Can you work these out from the model? Positions are in its coordinate system, mm. A direction names the side the tool comes from. Coordinates: 2 decimals unless noted, no trailing zeros. Write each loop counter-clockwise with the first axis right and the second up, starting at its lowest first coordinate (ties: lowest second). Pieces come first, ordered by that corner, then holes. Notation, with made-up numbers: (3, -22) -> (13, -22) arc R20 ccw to (13, 15) -> close; hole circle Ø3 at (76.5, 26). An arc over 180 degrees is marked (long way). Use one line per item in the form item = value.
```python
from build123d import *

# Parameters (mm, degrees)
F0_R     = 1.5
F1_DEPTH = 40
F2_DEPTH = 8
F4_D     = 4.4
F4_DEPTH = 9
F4_TIP   = 1.3218933619


with BuildPart() as f1:
    # F0 (on Top) → F1 (new body)
    with BuildSketch(Plane.XY):
        Polygon((4.0414518843, 0), (2.0207259422, 3.5), (-2.0207259422, 3.5), (-4.0414518843, 0), (-2.0207259422, -3.5), (2.0207259422, -3.5), align=None)
        Circle(F0_R, mode=Mode.SUBTRACT)
        Circle(F0_R)
    extrude(amount=F1_DEPTH)

    # F0 (on Top) → F2 (join)
    with BuildSketch(Plane.XY):
        Circle(F0_R)
    extrude(amount=-F2_DEPTH)

    # F4
    with Locations(Plane.XY.offset(40)):
        with Locations((0, 0)):
            Hole(F4_D / 2, depth=F4_DEPTH)
            with Locations((0, 0, -(F4_DEPTH + F4_TIP / 2))):  # 118° drill point
                Cone(0, F4_D / 2, F4_TIP, mode=Mode.SUBTRACT)


solid = f1.part
```
Q1. Will this pin go through, and if not, where does the flat tip stop? pin 1 (1 mm diameter, centred on y = 2.5, z = 18, fed in from -X).
Return value:
pin_1 = -2.89
Q2. If I drill on line 1 (Y direction, x = 0, z = 35.25); line 2 (X direction, y = 0, z = 37.75); line 3 (Z direction, x = -2, y = 1.75), over which ranges is the centre line in solid material (lowest first)? Write a range as from..to.
Return value:
line_1 = -3.5..-2.2, 2.2..3.5
line_2 = -4.04..-2.2, 2.2..4.04
line_3 = 0..40
Q3. Suppose I cut it at A-A (z = 30.5). Write out the boundary of the cut face in (x, y).
Return value:
outline = (-4.04, 0) -> (-2.02, -3.5) -> (2.02, -3.5) -> (4.04, 0) -> (2.02, 3.5) -> (-2.02, 3.5) -> close; hole circle Ø2.74 at (0, 0)
Q4. Thinking about a two-plate mould opening in X: for faces 1 (the conical face through (-0.083, -0.373, 29.908)), 2 (the cylindrical face through (-2.1, 0.66, 35.44)), 3 (the flat face through (0, -3.5, 20)), 4 (the flat face through (-3, 1.8, 19.7)), which applies, released by +X, released by -X, zero draft, split by the parting line, or undercut?
Return value:
face_1 = undercut
face_2 = undercut
face_3 = zero draft
face_4 = released by -X
Q5. Suppose I cut it at C-C (x = 3.25). Write out the boundary of the cut face in (y, z).
Return value:
outline = (-1.37, 0) -> (1.37, 0) -> (1.37, 40) -> (-1.37, 40) -> close
Q6. For faces 5 (the flat face through (2, 0, 0)), 6 (the flat face through (2, 2, 40)), which set-ups out of +Z, -Z, +X, -X, +Y, -Y let a thin tool reach every point of the face, with its end or its side?
Return value:
face_5 = -Z
face_6 = +Z, +X, -X, +Y, -Y
Q7. Suppose I cut it at B-B (z = 8). Write out the boundary of the cut face in (x, y).
Return value:
outline = (-4.04, 0) -> (-2.02, -3.5) -> (2.02, -3.5) -> (4.04, 0) -> (2.02, 3.5) -> (-2.02, 3.5) -> close
